```python
from build123d import *

# Parameters (mm, degrees)
SKETCH1_W           = 130
SKETCH1_H           = 65
BOSS_EXTRUDE1_DEPTH = 2
SKETCH2_W           = 130
SKETCH2_H           = 65
SKETCH2_W_2         = 126
SKETCH2_H_2         = 61
BOSS_EXTRUDE2_DEPTH = 120
SKETCH4_W           = 40
SKETCH4_H           = 1
SKETCH4_W_2         = 2
SKETCH4_H_2         = 19
SKETCH4_H_3         = 40
BOSS_EXTRUDE3_DEPTH = 120


with BuildPart() as part:
    # Sketch1 → Boss-Extrude1 (new body)
    with BuildSketch(Plane(origin=(0, 0, 0), x_dir=(1, 0, 0), z_dir=(0, 1, 0))):
        Rectangle(SKETCH1_W, SKETCH1_H)
    extrude(amount=BOSS_EXTRUDE1_DEPTH)

    # Sketch2 → Boss-Extrude2 (add)
    with BuildSketch(Plane(origin=(0, 2, 0), x_dir=(1, 0, 0), z_dir=(0, 1, 0))):
        Rectangle(SKETCH2_W, SKETCH2_H)
        Rectangle(SKETCH2_W_2, SKETCH2_H_2, mode=Mode.SUBTRACT)
    extrude(amount=BOSS_EXTRUDE2_DEPTH)

    # Sketch4 → Boss-Extrude3 (add)
    with BuildSketch(Plane(origin=(0, 2, 0), x_dir=(1, 0, 0), z_dir=(0, 1, 0))):
        Polygon((-21, 30.5), (-23, 30.5), (-23, 0.5), (-23, -0.5), (-23, -9.5), (-19, -9.5), (-19, 30.5), align=None)
        with Locations((-43, 0)):
            Rectangle(SKETCH4_W, SKETCH4_H)
        with Locations((-22, -21)):
            Rectangle(SKETCH4_W_2, SKETCH4_H_2)
        Polygon((11, -9.5), (-19, -9.5), (-23, -9.5), (-23, -11.5), (-21, -11.5), (13, -11.5), (13, -9.5), align=None)
        with Locations((12, 10.5)):
            Rectangle(SKETCH4_W_2, SKETCH4_H_3)
    extrude(amount=BOSS_EXTRUDE3_DEPTH)


solid = part.part
```
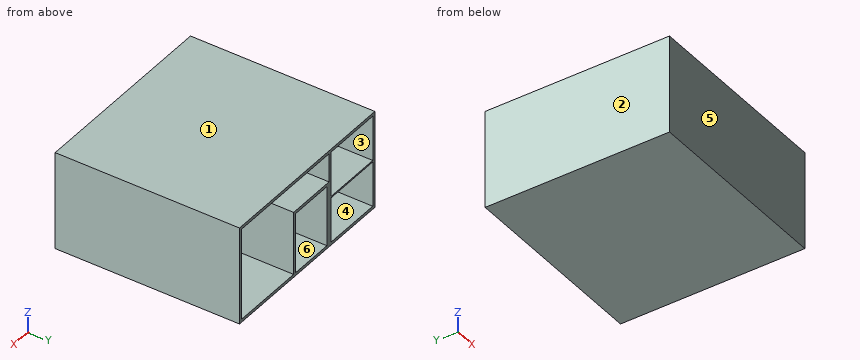
Part model, mm, in its own coordinate system. Face numbers are marked on the shaded views. A direction names the side the tool comes from. Coordinates: 2 decimals unless noted, no trailing zeros. Order: outer loops, then holes, each group sorted by start corner. A loop starts at its lowest first (then second) coordinate and runs counter-clockwise, first axis right, second up. Notation, with made-up numbers: (68.5, 85) - (112.5, 85) arc R9 ccw to (112.5, 92) - close; hole circle Ø2 at (83, 74.5). An arc over 180 degrees is marked (long way). Return JSON: item names as keys, results as strings. Group by question number.
Item 1: Drill centre lines: probe 1 along X at (y, z) = (97.5, -24); probe 2 along Z at (x, y) = (-50, 87); probe 3 along X at (y, z) = (115.5, 20). Where is each one in solid material? Low to high. Write a range as from..to.
Item 2: Which spindle directions (+Z, -Z, +X, -X, +Y, -Y) get a long thin tool onto all of the face, cutting with end or side? Do the marked faces 5 and 6. Say none if no direction does.
Item 3: Cut at B-B (z = -25). List the corners of the cut face in (x, y), plus the area to 3 significant figures.
Item 4: Pin check, flat tips, straight feed: pin 1 (1.5 mm diameter, centred on x = -20, z = 12, fed in from -Y); pin 2 (3 mm diameter, centred on x = 23, z = 1.5, fed in from +Y). Stop position of each tip, or through.
Item 5: Cut at C-C (x = 37.5). List the corners of the cut face in (y, z).
Item 6: Cut at D-D (z = 27). List the corners of the cut face in (x, y).
Item 7: Pull direction Z, two halves, no side cores. Call the marked faces 1, 2, 3 and 4: pulls with the +Z half, pulls with the -Z half, needs draft (parallel to the pull), parting line crosses it, or undercut.
Item 8: Cut at A-A (y = 106). List the corners of the cut face in (x, z), plus the area to 3 significant figures.
Check values:
{
 "1": {"probe 1": "x = -65..-63, -23..-19, 11..13, 63..65", "probe 2": "z = -32.5..-30.5, -0.5..0.5, 30.5..32.5", "probe 3": "x = -65..-63, -23..-21, 63..65"},
 "2": {"face 5": "+Z, -Z, +X, -X, -Y", "face 6": "+Y"},
 "3": {"outline": "(-65, 0) - (65, 0) - (65, 122) - (63, 122) - (63, 2) - (13, 2) - (13, 122) - (11, 122) - (11, 2) - (-19, 2) - (-19, 122) - (-23, 122) - (-23, 2) - (-63, 2) - (-63, 122) - (-65, 122) - close", "area": "1,460 mm2"},
 "4": {"pin 1": "stops at y = 0", "pin 2": "stops at y = 2"},
 "5": {"outline": "(0, -32.5) - (122, -32.5) - (122, -30.5) - (2, -30.5) - (2, 30.5) - (122, 30.5) - (122, 32.5) - (0, 32.5) - close"},
 "6": {"outline": "(-65, 0) - (65, 0) - (65, 122) - (63, 122) - (63, 2) - (-21, 2) - (-21, 122) - (-23, 122) - (-23, 2) - (-63, 2) - (-63, 122) - (-65, 122) - close"},
 "7": {"face 1": "pulls with the +Z half", "face 2": "needs draft", "face 3": "undercut", "face 4": "undercut"},
 "8": {"outline": "(-65, -32.5) - (65, -32.5) - (65, 32.5) - (-65, 32.5) - close; hole (-63, -30.5) - (-23, -30.5) - (-23, -0.5) - (-63, -0.5) - close; hole (-63, 0.5) - (-23, 0.5) - (-23, 30.5) - (-63, 30.5) - close; hole (-21, 11.5) - (13, 11.5) - (13, -30.5) - (63, -30.5) - (63, 30.5) - (-21, 30.5) - close; hole (-19, -30.5) - (11, -30.5) - (11, 9.5) - (-19, 9.5) - close", "area": "1,150 mm2"}
}
